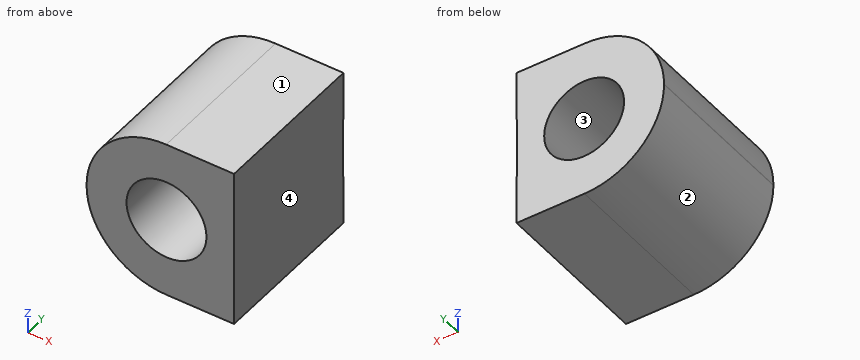
from build123d import *

# Parameters (mm, degrees)
SKETCH1_R           = 3.175
BOSS_EXTRUDE1_DEPTH = 12.7


with BuildPart() as part:
    # Sketch1 → Boss-Extrude1 (new body)
    with BuildSketch(Plane(origin=(0, 0, 0), x_dir=(1, 0, 0), z_dir=(0, 1, 0))):
        with BuildLine():
            Line((-0.0254, -6.35), (5.366129104, -6.35))
            ThreePointArc((5.366129104, -6.35), (5.35, 0), (5.366129104, 6.35))
            Line((5.366129104, 6.35), (-0.0254, 6.35))
            ThreePointArc((-0.0254, 6.35), (-4.497567548, 4.497567548), (-6.35, 0.0254))
            Line((-6.35, 0.0254), (-6.35, -0.0254))
            ThreePointArc((-6.35, -0.0254), (-4.497567548, -4.497567548), (-0.0254, -6.35))
        make_face()
        Circle(SKETCH1_R, mode=Mode.SUBTRACT)
    extrude(amount=BOSS_EXTRUDE1_DEPTH)


solid = part.part
Verification items for the finished model (mm, model axes). Face numbers are marked on the shaded views. Give positions to 0.01 mm unless a question says otherwise; leave off trailing zeros. Order: outer loops, then holes, each group sorted by start corner. A loop starts at its lowest first (then second) coordinate and runs counter-clockwise, first axis right, second up. Notation, with made-up numbers: (8, 34.25) -> (65, 34.25) arc R26 ccw to (65, 61.25) -> close; hole circle Ø10 at (46.25, -7.75). An arc over 180 degrees is marked (long way). Answer as CSV lines item,"result".
Q1. Scan lines: probe 1 along X at (y, z) = (8.5, 0) (3 decimals); probe 2 along Z at (x, y) = (0, 8.5) (3 decimals); probe 3 along Z at (x, y) = (-2.5, 5.5). Record each from-to range of solid material in increasing order.
Solutions:
probe 1,"x = -6.35 to -3.175, 3.175 to 5.35"
probe 2,"z = -6.35 to -3.175, 3.175 to 6.35"
probe 3,"z = -5.85 to -1.96, 1.96 to 5.85"
Q2. Sectioned sample at A-A on z = -2.25. Record the cut outline in (x, y), plus the area to 3 significant figures.
Solutions:
outline,"(-5.95, 0) -> (-2.24, 0) -> (-2.24, 12.7) -> (-5.95, 12.7) -> close; (2.24, 0) -> (5.35, 0) -> (5.35, 12.7) -> (2.24, 12.7) -> close"
area,"86.6 mm²"
Q3. Release check for a two-part mould opening along Z. For the marked faces 1, 2, 3 and 4 record: +Z half, -Z half, draft (parallel to the pull), parting line (faces both ways), or undercut.
Solutions:
face 1,"+Z half"
face 2,"-Z half"
face 3,"undercut"
face 4,"undercut"
Q4. Depth check by flat-ended pin: pin 1 (5 mm diameter, centred on y = 8.5, z = -4.5, fed in from -X); pin 2 (1.5 mm diameter, centred on y = 2, z = -2.5, fed in from +X). Enter the tip coordinate at first touch or a pass-through.
Solutions:
pin 1,"stops at x = -6.03"
pin 2,"stops at x = 5.35"
Q5. Sectioned sample at C-C on z = -4.25. Record the cut outline in (x, y).
Solutions:
outline,"(-4.73, 0) -> (5.36, 0) -> (5.36, 12.7) -> (-4.73, 12.7) -> close"
Q6. Sectioned sample at B-B on x = -3. Record the cut outline in (y, z), plus the area to 3 significant figures.
Solutions:
outline,"(0, -5.61) -> (12.7, -5.61) -> (12.7, -1.04) -> (0, -1.04) -> close; (0, 1.04) -> (12.7, 1.04) -> (12.7, 5.61) -> (0, 5.61) -> close"
area,"116 mm²"
